Verification items for the finished model (mm, model axes). Face numbers are marked on the shaded views. Give positions to 0.01 mm unless a question says otherwise; leave off trailing zeros. Order: outer loops, then holes, each group sorted by start corner. A loop starts at its lowest first (then second) coordinate and runs counter-clockwise, first axis right, second up.
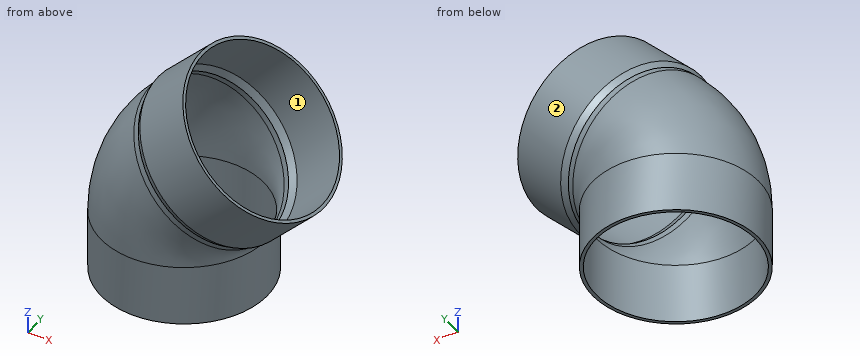
Autodesk Inventor part; units mm, degrees
ref_plane "YZ Plane" through (0, 0, 0) normal (1, 0, 0) x (0, 1, 0)
ref_plane "XZ Plane" through (0, 0, 0) normal (0, 1, 0) x (-1, 0, 0)
ref_plane "XY Plane" through (0, 0, 0) normal (0, 0, 1) x (1, 0, 0)
sketch "Sketch1" plane through (0, 0, 0) normal (0, 1, 0) x (-1, 0, 0)
  line L0 (0, 0) -> (0, 58)
  line L1 (0, 0) -> (76.8, 0) construction
  line L2 (76.8, 0) -> (76.8, 58)
  line L3 (76.8, 58) -> (80, 58)
  line L4 (80, 58) -> (80, 0)
  line L5 (80, 0) -> (76.8, 0)
  line L6 (0, 58) -> (76.8, 58) construction
  dimension "d0" = 3.2
  dimension "d1" = 58
  dimension "d2" = 160
revolve "Revolution1" add sketch "Sketch1" angle 360 about axis through (0, 0, 0) along (0, 0, 1)
sketch "Sketch2" plane through (0, 0, 0) normal (0, 1, 0) x (-1, 0, 0)
  line L0 (0, 94) -> (-29.6985, 123.6985) construction
  line L1 (-29.6985, 123.6985) -> (-75.7477, 169.7477) construction
  line L2 (-75.7477, 169.7477) -> (-19.0023, 226.493) construction
  line L3 (-19.0023, 226.493) -> (-16.9659, 228.5294)
  line L4 (-16.9659, 228.5294) -> (24.5135, 187.05)
  line L5 (24.5135, 187.05) -> (26.8701, 180.267)
  line L6 (26.8701, 180.267) -> (24.6073, 178.0043)
  line L7 (24.6073, 178.0043) -> (22.0099, 185.4808)
  line L8 (22.0099, 185.4808) -> (-19.0023, 226.493)
  line L9 (22.0099, 185.4808) -> (-34.7355, 128.7355) construction
  line L10 (-29.6985, 123.6985) -> (24.6073, 178.0043) construction
  line L11 (-29.6985, 123.6985) -> (-25.4558, 119.4558)
  line L12 (-80, 58) -> (80, 58)
  line L13 (0, 94) -> (0, 58) construction
  arc A0 (0, 58) -> (-25.4558, 119.4558) centre (-86.9117, 58) ccw
  dimension "d5" = 160.5
  dimension "d6" = 2.88
  dimension "d7" = 58
  dimension "d8" = 160
  dimension "d9" = 3.2
  dimension "d10" = 42
  dimension "d11" = 2.88
  dimension "d12" = 45
  dimension "d13" = 36
sketch "Sketch3" plane through (0, 0, 58) normal (0, 0, 1) x (1, 0, 0)
  circle A0 centre (0, 0) radius 76.8
  circle A1 centre (0, 0) radius 80
  circle A2 centre (0, 0) radius 80
  circle A3 centre (0, 0) radius 76.8
sweep "Sweep1" add profiles "Sketch3" path "Sketch2" path curves A0 L11
revolve "Revolution2" add sketch "Sketch2" angle 360 about axis through (29.6985, 0, 123.6985) along (0.7071068, 0, 0.7071068)
equation "\"d5\" = Ds"
equation "\"d6\" = e2"
equation "\"d7\" = L1"
equation "\"d8\" = De"
equation "\"d9\" = e"
equation "\"d10\" = z2"
equation "\"d11\" = e2"
equation "\"d13\" = z1"
equation "\"d0\" = e"
equation "\"d1\" = L1"
equation "\"d2\" = De"
equation "\"z1\" = 36"
equation "\"L1\" = 58"
equation "\"De\" = 160"
equation "\"e\" = 3.2"
equation "\"z2\" = 42"
equation "\"Ds\" = 160.5"
equation "\"e2\" = 0.9 * e"
equation "\"e3\" = 0.75 * e"
equation "\"Size_Designation\" = 1.2345"
properties part number "ISO 3633 45 Deg Bend with Single Socket for Cemented Type Joints DN160" material "PVC, Unplasticized"
(1) Go/stop test with flat-tipped pins: pin 1 (1.5 mm diameter, centred on x = -13.5, z = 135, fed in from +Y); pin 2 (8 mm diameter, centred on y = -3.5, z = 46, fed in from +X); pin 3 (4 mm diameter, centred on x = 18.5, z = 58, fed in from +Y). Record where each tip stops, or that it passes through.
Solved:
pin 1: stops at y = 69.92
pin 2: stops at x = 80
pin 3: stops at y = 78.28
(2) Section check A-A, the plane z = 28. Enter the section's corners in (x, y), then the cut area to 3 significant figures.
Solved:
outline: circle Ø160 at (0, 0); hole circle Ø153.6 at (0, 0)
area: 1,580 mm2
(3) Release check for a two-part mould opening along X. For the marked faces 1 and 2 record: pulls with the +X half, pulls with the -X half, needs draft (parallel to the pull), parting line crosses it, or undercut.
Solved:
face 1: undercut
face 2: parting line crosses it
(4) Scan lines: line 1 (X direction, y = 0, z = 44); line 2 (Y direction, x = -34, z = 146). Record each from-to range of solid material in increasing order.
Solved:
line 1: x = -80 to -76.8, 76.8 to 80
line 2: y = -49.77 to -44.44, 44.44 to 49.77
